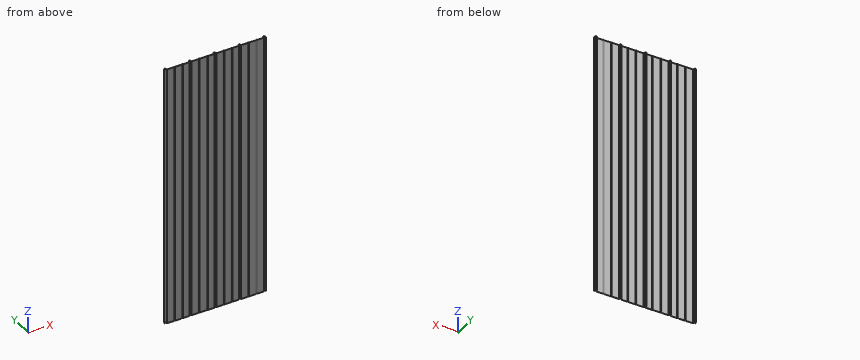
from build123d import *

# Parameters (mm, degrees)
SKETCH1_W           = 4.7625
SKETCH1_H           = 0.508
SKETCH1_W_2         = 31.504412895
BOSS_EXTRUDE1_DEPTH = 2438.4
LPATTERN1_COUNT     = 4
LPATTERN1_PITCH     = 228.6


with BuildPart() as part:
    # Sketch1 → Boss-Extrude1 (new body)
    with BuildSketch(Plane.XY):
        Polygon((4.7625, 15.875), (5.2705, 15.875), (5.2705, 18.542), (9.525, 18.542), (9.525, 19.05), (4.7625, 19.05), align=None)
        with BuildLine():
            ThreePointArc((5.249075753, 15.729027274), (5.265115401, 15.801231722), (5.2705, 15.875))
            Line((5.2705, 15.875), (4.7625, 15.875))
            Line((4.7625, 15.875), (0, 0))
            Line((0, 0), (-0.1524, -0.508))
            Line((-0.1524, -0.508), (0.377967571, -0.508))
            Line((0.377967571, -0.508), (0.486575753, -0.145972726))
            Line((0.486575753, -0.145972726), (5.249075753, 15.729027274))
        make_face()
        Polygon((9.525, 19.05), (9.525, 18.542), (13.7795, 18.542), (13.7795, 15.875), (14.2875, 15.875), (14.2875, 19.05), align=None)
        Polygon((14.2875, 15.875), (13.7795, 15.875), (13.800924247, 15.729027274), (18.519632429, 0), (19.05, 0), align=None)
        Polygon((79.129412895, 0), (19.05, 0), (18.519632429, 0), (18.563424247, -0.145972726), (18.672032429, -0.508), (79.129412895, -0.508), align=None)
        Polygon((79.422706832, 0), (79.129412895, 0), (79.129412895, -0.508), align=None)
        Polygon((80.9625, 3.175), (79.129412895, 0), (79.422706832, 0), (80.9625, 2.667), align=None)
        with Locations((83.34375, 2.921)):
            Rectangle(SKETCH1_W, SKETCH1_H)
        Polygon((92.320587105, -0.508), (92.320587105, 0), (92.027293168, 0), align=None)
        Polygon((92.320587105, 0), (90.4875, 3.175), (90.4875, 2.667), (92.027293168, 0), align=None)
        with Locations((88.10625, 2.921)):
            Rectangle(SKETCH1_W, SKETCH1_H)
        with Locations((108.072793553, -0.254)):
            Rectangle(SKETCH1_W_2, SKETCH1_H)
        with Locations((139.577206448, -0.254)):
            Rectangle(SKETCH1_W_2, SKETCH1_H)
        Polygon((155.622706832, 0), (155.329412895, 0), (155.329412895, -0.508), align=None)
        Polygon((157.1625, 3.175), (155.329412895, 0), (155.622706832, 0), (157.1625, 2.667), align=None)
        with Locations((159.54375, 2.921)):
            Rectangle(SKETCH1_W, SKETCH1_H)
        with Locations((164.30625, 2.921)):
            Rectangle(SKETCH1_W, SKETCH1_H)
        Polygon((168.520587105, 0), (166.6875, 3.175), (166.6875, 2.667), (168.227293168, 0), align=None)
        Polygon((168.520587105, -0.508), (168.520587105, 0), (168.227293168, 0), align=None)
        Polygon((228.6, 0), (168.520587105, 0), (168.520587105, -0.508), (228.977967571, -0.508), (229.086575753, -0.145972726), (229.130367571, 0), align=None)
        Polygon((233.3625, 15.875), (228.6, 0), (229.130367571, 0), (233.849075753, 15.729027274), (233.8705, 15.875), align=None)
        Polygon((233.3625, 19.05), (233.3625, 15.875), (233.8705, 15.875), (233.8705, 18.542), (238.125, 18.542), (238.125, 19.05), align=None)
        Polygon((242.8875, 19.05), (238.125, 19.05), (238.125, 18.542), (242.3795, 18.542), (242.3795, 15.875), (242.8875, 15.875), align=None)
        Polygon((247.163424247, -0.145972726), (247.272032429, -0.508), (247.8024, -0.508), (247.65, 0), (242.8875, 15.875), (242.3795, 15.875), (242.400924247, 15.729027274), align=None)
    boss_extrude1 = extrude(amount=BOSS_EXTRUDE1_DEPTH)

    # LPattern1: Boss-Extrude1 ×4
    with Locations(*[(i * LPATTERN1_PITCH, 0, 0) for i in range(1, LPATTERN1_COUNT)]):
        add(boss_extrude1)


solid = part.part
Work out the finished part from the listing and answer in its coordinate system (mm). Give positions to 0.01 mm unless a question says otherwise; leave off trailing zeros. Loops run counter-clockwise (first coordinate to the right, second up) from the corner with the lowest first, then second, coordinate; pieces in that order, holes last. Notation, with made-up numbers: (14.25, 13) - (31.25, 13) arc R23 ccw to (31.25, 50) - close; hole circle Ø9 at (21, 37.25). An arc over 180 degrees is marked (long way). Answer in a Markdown table with one row per item. Add a question column.
Q1. The part is cut by section B-B (y = 12). State how many separate pieces and enclosed holes the cut face has, and give its area (3 significant figures).
Q2. Each of these flat-tipped pins is pushed along its axis until it touches: P1, Ø2.5, axis at y = 17, z = 1418, coming from the +X side (3 decimals); P2, Ø12, axis at x = 271, z = 766, coming from the +Y side; P3, Ø5, axis at x = 87.5, z = 919, coming from the +Y side (3 decimals). Where does it stop, or does it pass through?
Q3. The part is cut by section A-A (x = 732). Determine the outline of the cut face in (y, z).
Q4. Consider line 1 along Y through (x, z) = (319, 731.5) (3 decimals); line 2 along Y through (x, z) = (235.5, 900). Determine where each line is inside the solid, lowest interval first.
Solution:
| question | item | result |
|---|---|---|
| 1 | separate pieces | 10 |
| 1 | enclosed holes | 0 |
| 1 | area | 12,900 mm² |
| 2 | P1 | stops at x = 928.725 |
| 2 | P2 | stops at y = 0 |
| 2 | P3 | stops at y = 3.175 |
| 3 | outline | (-0.51, 0) - (0, 0) - (0, 2438.4) - (-0.51, 2438.4) - close |
| 4 | line 1 | y = 2.667 to 3.175 |
| 4 | line 2 | y = 18.54 to 19.05 |
